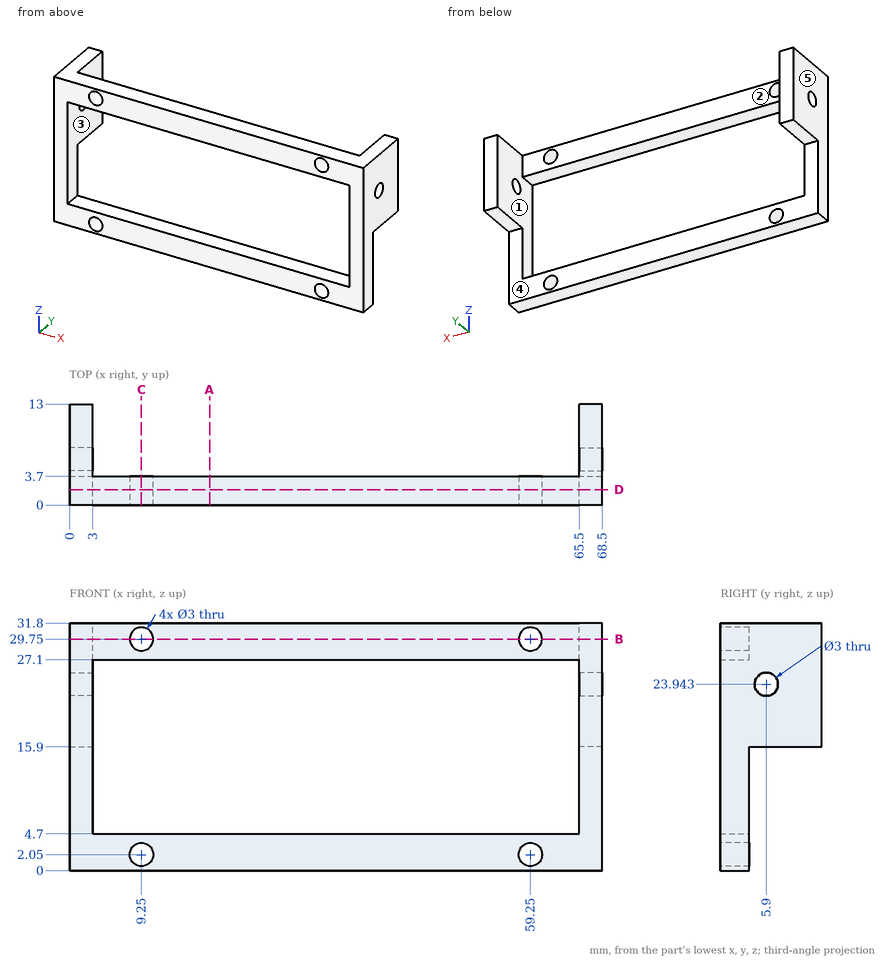
Design review of the part shown in the three views and the two pictorial views. Dimensions are in mm from the part's minimum x, y and z. A direction names the side the tool comes from. Round coordinates to 2 decimals unless told otherwise and drop trailing zeros. Loops run counter-clockwise (first coordinate to the right, second up) from the corner with the lowest first, then second, coordinate; pieces in that order, holes last.
Q1. Add section C-C on x = 9.25. Write out the cut boundary in (y, z), plus the area to 3 significant figures.
Result sheet:
outline: (0, 0) - (3.7, 0) - (3.7, 0.55) - (0, 0.55) - close; (0, 3.55) - (3.7, 3.55) - (3.7, 4.7) - (0, 4.7) - close; (0, 27.1) - (3.7, 27.1) - (3.7, 28.25) - (0, 28.25) - close; (0, 31.25) - (3.7, 31.25) - (3.7, 31.8) - (0, 31.8) - close
area: 12.6 mm2
Q2. Machinability: for the marked faces 3, 4 and 5, which of the approach directions +Z, -Z, +X, -X, +Y, -Y give a long, thin tool a straight path to every point of the face, cutting with its end or side? Answer none if there is none.
Result sheet:
face 3: +Y
face 4: -Z, +X, -X, +Y
face 5: +Z, -Z, -X, +Y, -Y
Q3. Insertion check: pin 1 Ø8 at (x, z) = (23.5, 7.5) entering from +Y; pin 2 Ø2.5 at (x, y) = (66.5, 7) entering from -Z. Each pin has a flat end and moves straight along its axis. Give the tip position at first contact, or say it passes through.
Result sheet:
pin 1: stops at y = 3.7
pin 2: stops at z = 15.9
Q4. Mouldability with a two-part tool opening along Z and no side actions: class the marked faces 1 and 2 as +Z half, -Z half, draft (parallel to the pull), parting line (faces both ways), or undercut.
Result sheet:
face 1: undercut
face 2: draft
Q5. Add section D-D on y = 2. Write out the cut boundary in (x, z).
Result sheet:
outline: (0, 0) - (68.5, 0) - (68.5, 31.8) - (0, 31.8) - close; hole (3, 4.7) - (65.5, 4.7) - (65.5, 27.1) - (3, 27.1) - close; hole circle Ø3 at (9.25, 2.05); hole circle Ø3 at (9.25, 29.75); hole circle Ø3 at (59.25, 2.05); hole circle Ø3 at (59.25, 29.75)
Q6. To check wall thickness, follow line 1 along Z through (x, y) = (9.25, 2.8); line 2 along Z through (x, y) = (66.85, 5.9); line 3 along X through (y, z) = (1.75, 22.5). State the ranges of each line that lie inside material, in increasing order.
Result sheet:
line 1: z = 0 to 0.55, 3.55 to 4.7, 27.1 to 28.25, 31.25 to 31.8
line 2: z = 15.9 to 22.44, 25.44 to 31.8
line 3: x = 0 to 3, 65.5 to 68.5
Q7. Add section A-A on x = 18. Write out the cut boundary in (y, z).
Result sheet:
outline: (0, 0) - (3.7, 0) - (3.7, 4.7) - (0, 4.7) - close; (0, 27.1) - (3.7, 27.1) - (3.7, 31.8) - (0, 31.8) - close
Q8. Add section B-B on z = 29.75. Write out the cut boundary in (x, y).
Result sheet:
outline: (0, 0) - (7.75, 0) - (7.75, 3.7) - (3, 3.7) - (3, 13) - (0, 13) - close; (10.75, 0) - (57.75, 0) - (57.75, 3.7) - (10.75, 3.7) - close; (60.75, 0) - (68.5, 0) - (68.5, 13) - (65.5, 13) - (65.5, 3.7) - (60.75, 3.7) - close
